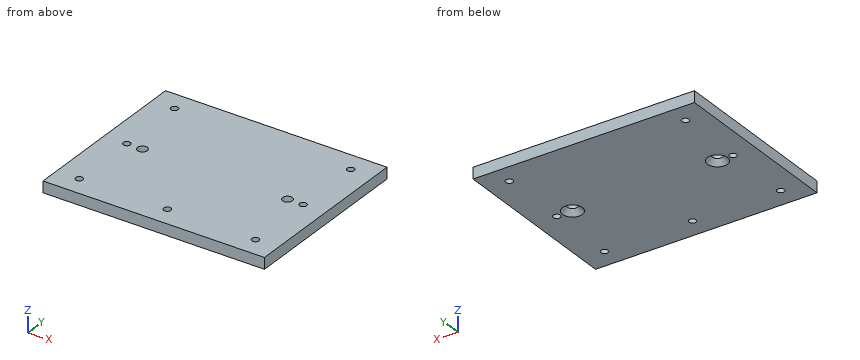
```python
from build123d import *

# Parameters (mm, degrees)
F0_W           = 99.5
F0_H           = 80.4
F1_DEPTH       = 5.08
F3_D           = 4.4
F3_DEPTH       = 38.1
F3_CSINK_D     = 8.96
F3_CSINK_ANGLE = 90
F3_TIP         = 1.3218933619
F5_D           = 3.2
F5_DEPTH       = 37.175
F5_TIP         = 0.9613769904


# Not quite as in the source:
# - a feature names something its author has since deleted; it is built from what else it names


with BuildPart() as f1:
    # F0 (on Top) → F1 (new body)
    with BuildSketch(Plane.XY):
        Rectangle(F0_W, F0_H)
    extrude(amount=F1_DEPTH)

    # F3
    with Locations(Plane(origin=(0, 0, 0), x_dir=(1, 0, 0), z_dir=(0, 0, -1))):
        with Locations((-32.5796, 0), (32.5796, 0)):
            CounterSinkHole(F3_D / 2, F3_CSINK_D / 2, depth=F3_DEPTH, counter_sink_angle=F3_CSINK_ANGLE)
            with Locations((0, 0, -(F3_DEPTH + F3_TIP / 2))):  # 118° drill point
                Cone(0, F3_D / 2, F3_TIP, mode=Mode.SUBTRACT)

    # F5
    with Locations(Plane(origin=(0, 0, 0), x_dir=(1, 0, 0), z_dir=(0, 0, -1))):
        with Locations((-39.59, 31.242), (-39.59, 0), (-39.59, -31.242), (39.59, -31.242), (39.59, 0), (39.59, 31.242), (0, 31.242)):
            Hole(F5_D / 2, depth=F5_DEPTH)
            with Locations((0, 0, -(F5_DEPTH + F5_TIP / 2))):  # 118° drill point
                Cone(0, F5_D / 2, F5_TIP, mode=Mode.SUBTRACT)


solid = f1.part
```
Can you work these out from the model? Positions are in its coordinate system, mm. Round coordinates to 2 decimals unless told otherwise and drop trailing zeros. Loops run counter-clockwise (first coordinate to the right, second up) from the corner with the lowest first, then second, coordinate; pieces in that order, holes last. Notation, with made-up numbers: (28.25, 34.5) -> (47.25, 34.5) arc R18 ccw to (47.25, 51.5) -> close; hole circle Ø7 at (54.5, 7). An arc over 180 degrees is marked (long way). Answer in a Markdown table with one row per item.
Item 1: Suppose I cut it at A-A, the plane y = 0. List the corners of the cut face in (x, z) for me, plus the area to 3 significant figures.
Answer block:
| item | result |
|---|---|
| outline | (-49.75, 0) -> (-41.19, 0) -> (-41.19, 5.08) -> (-49.75, 5.08) -> close; (-37.99, 0) -> (-37.06, 0) -> (-34.78, 2.28) -> (-34.78, 5.08) -> (-37.99, 5.08) -> close; (-30.38, 2.28) -> (-28.1, 0) -> (28.1, 0) -> (30.38, 2.28) -> (30.38, 5.08) -> (-30.38, 5.08) -> close; (34.78, 2.28) -> (37.06, 0) -> (37.99, 0) -> (37.99, 5.08) -> (34.78, 5.08) -> close; (41.19, 0) -> (49.75, 0) -> (49.75, 5.08) -> (41.19, 5.08) -> close |
| area | 418 mm² |
Item 2: If I drill on probe 1 along Y at (x, z) = (-39.59, 3.8); probe 2 along X at (y, z) = (1, 2.8); probe 3 along X at (y, z) = (-2, 2), over which ranges is the centre line in solid material (lowest first)?
Answer block:
| item | result |
|---|---|
| probe 1 | -40.2 to -32.84, -29.64 to -1.6, 1.6 to 29.64, 32.84 to 40.2 |
| probe 2 | -49.75 to -40.84, -38.34 to -34.54, -30.62 to 30.62, 34.54 to 38.34, 40.84 to 49.75 |
| probe 3 | -49.75 to -34.05, -31.11 to 31.11, 34.05 to 49.75 |
Item 3: Suppose I cut it at B-B, the plane x = 39.59. List the corners of the cut face in (y, z) for me.
Answer block:
| item | result |
|---|---|
| outline | (-40.2, 0) -> (-32.84, 0) -> (-32.84, 5.08) -> (-40.2, 5.08) -> close; (-29.64, 0) -> (-1.6, 0) -> (-1.6, 5.08) -> (-29.64, 5.08) -> close; (1.6, 0) -> (29.64, 0) -> (29.64, 5.08) -> (1.6, 5.08) -> close; (32.84, 0) -> (40.2, 0) -> (40.2, 5.08) -> (32.84, 5.08) -> close |
Item 4: Suppose I cut it at C-C, the plane x = 0. List the corners of the cut face in (y, z) for me.
Answer block:
| item | result |
|---|---|
| outline | (-40.2, 0) -> (-32.84, 0) -> (-32.84, 5.08) -> (-40.2, 5.08) -> close; (-29.64, 0) -> (40.2, 0) -> (40.2, 5.08) -> (-29.64, 5.08) -> close |
